Autodesk Inventor part; units mm, degrees
ref_plane "YZ Plane" through (0, 0, 0) normal (1, 0, 0) x (0, 1, 0)
ref_plane "XZ Plane" through (0, 0, 0) normal (0, 1, 0) x (-1, 0, 0)
ref_plane "XY Plane" through (0, 0, 0) normal (0, 0, 1) x (1, 0, 0)
ref_plane "Arbeitsebene1" through (0, 0, 0) normal (0, 0, 1) x (1, 0, 0)
sketch "Skizze1" plane through (0, 0, 0) normal (0, 0, 1) x (1, 0, 0)
  line L0 (0, 0) -> (40, 0)
  line L1 (40, 0) -> (40, 42)
  line L2 (0, 42) -> (40, 42)
  line L3 (0, 0) -> (0, 42)
  line L4 (5, 42) -> (35, 42)
  line L5 (40, 37) -> (40, 5)
  line L6 (35, 0) -> (5, 0)
  line L7 (0, 5) -> (0, 37)
  line L8 (0, 42) -> (40, 0) construction
  line L9 (40, 42) -> (0, 0) construction
  arc A0 (5, 42) -> (0, 37) centre (5, 37) ccw
  arc A1 (40, 37) -> (35, 42) centre (35, 37) ccw
  arc A2 (35, 0) -> (40, 5) centre (35, 5) ccw
  arc A3 (0, 5) -> (5, 0) centre (5, 5) ccw
  point P0 (20, 21)
  dimension "d0" = 5
extrude "Extrusion1" add sketch "Skizze1" along normal blind 10 contours A3 L3 A0 L2 A1 L1 A2 L0
sketch "Skizze2" plane through (0, 0, 10) normal (0, 0, 1) x (1, 0, 0)
  line L0 (0, 37) -> (0, 5)
  arc A0 (0, 5) -> (5, 0) centre (5, 5) ccw
  line L1 (5, 0) -> (35, 0)
  arc A1 (35, 0) -> (40, 5) centre (35, 5) ccw
  line L2 (40, 5) -> (40, 37)
  arc A2 (40, 37) -> (35, 42) centre (35, 37) ccw
  line L3 (35, 42) -> (5, 42)
  arc A3 (5, 42) -> (0, 37) centre (5, 37) ccw
  circle A4 centre (20, 21) radius 18.75
  point P0 (0, 0)
  dimension "d3" = 37.5
extrude "Extrusion2" cut sketch "Skizze2" against normal through all contours A4
sketch "Skizze3" plane through (0, 0, 10) normal (0, 0, 1) x (1, 0, 0)
  circle A0 centre (20, 21) radius 18.75
  line L0 (0, 37) -> (0, 5)
  arc A1 (0, 5) -> (5, 0) centre (5, 5) ccw
  line L1 (5, 0) -> (35, 0)
  arc A2 (35, 0) -> (40, 5) centre (35, 5) ccw
  line L2 (40, 5) -> (40, 37)
  arc A3 (40, 37) -> (35, 42) centre (35, 37) ccw
  line L3 (35, 42) -> (5, 42)
  arc A4 (5, 42) -> (0, 37) centre (5, 37) ccw
  circle A5 centre (5, 37) radius 1
  circle A6 centre (35, 37) radius 1
  circle A7 centre (35, 5) radius 1
  circle A8 centre (5, 5) radius 1
  point P0 (0, 0)
  dimension "d6" = 2
  dimension "d7" = 2
  dimension "d8" = 2
  dimension "d9" = 2
extrude "Extrusion3" cut sketch "Skizze3" against normal through all contours A5 | A6 | A7 | A8
properties part number "02_Coolingfan"
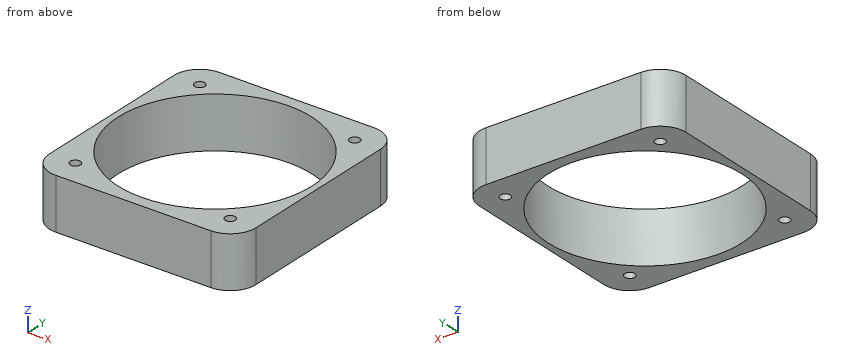
Geometry check sheet. Reference: the model listing, model coordinates, mm. Coordinates: 2 decimals unless noted, no trailing zeros. Order: outer loops, then holes, each group sorted by start corner. A loop starts at its lowest first (then second) coordinate and runs counter-clockwise, first axis right, second up. Notation, with made-up numbers: (34, 85.5) - (86, 85.5) arc R18 ccw to (86, 93.5) - close; hole circle Ø9 at (85, 49.25). An arc over 180 degrees is marked (long way). Answer in a Markdown table with one row per item. Add a question column.
1) Cross-section at B-B, the plane y = 21. Record the cut outline in (x, z), then the cut area to 3 significant figures.
2) Material ranges on line 1 along Y through (x, z) = (20, 3.5); line 2 along Y through (x, z) = (35, 1); line 3 along Y through (x, z) = (4.5, 7.75), recorded low to high. Write a range as [from, to].
3) Cross-section at C-C, the plane x = 21.5. Record the cut outline in (y, z), then the cut area to 3 significant figures.
4) Gauge pin test, flat end, axial feed: P1, Ø2.5, axis at x = 5, y = 5, coming from the +Z side. Record the tip position at first contact, or that the pin passes through.
5) Cross-section at A-A, the plane z = 4. Record the cut outline in (x, y), then the cut area to 3 significant figures.
Check result:
| question | item | result |
|---|---|---|
| 1 | outline | (0, 0) - (1.25, 0) - (1.25, 10) - (0, 10) - close; (38.75, 0) - (40, 0) - (40, 10) - (38.75, 10) - close |
| 1 | area | 25.0 mm² |
| 2 | line 1 | y = [0, 2.25], [39.75, 42] |
| 2 | line 2 | y = [0, 4], [6, 9.75], [32.25, 36], [38, 42] |
| 2 | line 3 | y = [0.03, 4.13], [5.87, 10.45], [31.55, 36.13], [37.87, 41.97] |
| 3 | outline | (0, 0) - (2.31, 0) - (2.31, 10) - (0, 10) - close; (39.69, 0) - (42, 0) - (42, 10) - (39.69, 10) - close |
| 3 | area | 46.2 mm² |
| 4 | P1 | stops at z = 10 |
| 5 | outline | (0, 5) arc R5 ccw to (5, 0) - (35, 0) arc R5 ccw to (40, 5) - (40, 37) arc R5 ccw to (35, 42) - (5, 42) arc R5 ccw to (0, 37) - close; hole circle Ø37.5 at (20, 21); hole circle Ø2 at (5, 5); hole circle Ø2 at (5, 37); hole circle Ø2 at (35, 5); hole circle Ø2 at (35, 37) |
| 5 | area | 542 mm² |
